from build123d import *

# Parameters (mm, degrees)
BOSS_EXTRUDE1_DEPTH  = 3
M3_CLEARANCE_HOLE1_D = 3.4
CUT_EXTRUDE1_DEPTH   = 10


with BuildPart() as part:
    # Sketch1 → Boss-Extrude1 (new body)
    with BuildSketch(Plane.XY):
        with BuildLine():
            Line((-93.536600288, 73.798841742), (22.52665856, 73.798841742))
            ThreePointArc((22.52665856, 73.798841742), (29.597726372, 76.72777393), (32.52665856, 83.798841742))
            Line((32.52665856, 83.798841742), (32.52665856, 133.798841742))
            ThreePointArc((32.52665856, 133.798841742), (29.597726372, 140.869909554), (22.52665856, 143.798841742))
            Line((22.52665856, 143.798841742), (-93.536600288, 143.798841742))
            ThreePointArc((-93.536600288, 143.798841742), (-100.6076681, 140.869909554), (-103.536600288, 133.798841742))
            Line((-103.536600288, 133.798841742), (-103.536600288, 83.798841742))
            ThreePointArc((-103.536600288, 83.798841742), (-100.6076681, 76.72777393), (-93.536600288, 73.798841742))
        make_face()
        Polygon((7.241251279, 79.113754803), (7.241251279, 115.298841742), (25.200464445, 115.298841742), (25.200464445, 141.298841742), (-63.686125174, 141.298841742), (-63.686125174, 139.298841742), (-98, 139.298841742), (-98, 79.113754803), align=None, mode=Mode.SUBTRACT)
    extrude(amount=BOSS_EXTRUDE1_DEPTH)

    # M3 Clearance Hole1 (through all)
    with Locations(Plane(origin=(0, 0, 0), x_dir=(-1, 0, 0), z_dir=(0, 0, -1))):
        with Locations((-28.497536526, 136.798841742), (-28.497536526, 81.798841742)):
            Hole(M3_CLEARANCE_HOLE1_D / 2)

    # Sketch2 → Cut-Extrude1 (cut)
    with BuildSketch(Plane.XY.offset(3)):
        with BuildLine():
            Line((-98, 111.232980273), (-100.276015927, 111.232980273))
            Line((-100.276015927, 111.232980273), (-100.276015927, 110.181279495))
            ThreePointArc((-100.276015927, 110.181279495), (-100.885260547, 108.11074669), (-101.110575194, 110.257259772))
            Line((-101.110575194, 110.257259772), (-101.110575194, 111.232980273))
            Line((-101.110575194, 111.232980273), (-103.536600288, 111.232980273))
            Line((-103.536600288, 111.232980273), (-103.536600288, 155.169137996))
            Line((-103.536600288, 155.169137996), (37.520914888, 146.495442913))
            Line((37.520914888, 146.495442913), (36.419995989, 128.591552724))
            Line((36.419995989, 128.591552724), (32.52665856, 128.591552724))
            Line((32.52665856, 128.591552724), (29.357018022, 128.591552724))
            Line((29.357018022, 128.591552724), (29.357018022, 126.79555932))
            ThreePointArc((29.357018022, 126.79555932), (28.609769319, 124.402587901), (28.09640217, 126.856390462))
            Line((28.09640217, 126.856390462), (28.09640217, 128.591552724))
            Line((28.09640217, 128.591552724), (25.200464445, 128.591552724))
            Line((25.200464445, 128.591552724), (-98, 111.232980273))
        make_face()
    extrude(amount=-CUT_EXTRUDE1_DEPTH, mode=Mode.SUBTRACT)


solid = part.part
Input: part model. Units: mm. Frame: model coordinates. A direction names the side the tool comes from. Give positions to 0.01 mm unless a question says otherwise; leave off trailing zeros. Write each loop counter-clockwise with the first axis right and the second up, starting at its lowest first coordinate (ties: lowest second). Pieces come first, ordered by that corner, then holes.
Q1. Set-up query: faces 1 (the face through (-103.537, 98, 1)), 2 (the face through (-99, 111.233, 2)), 3 (the face through (-46, 79.114, 1)). Return all of +Z, -Z, +X, -X, +Y, -Y with unobstructed straight access to the full face (end or side cutting, diameter ignored); none if empty.
Q2. First-contact query: P1, Ø0.5, axis at y = 127, z = 2, coming from the -X side; P2, Ø0.7, axis at x = -99, z = 1.5, coming from the +Y side. Flat tips, straight axial feed; report the tip coordinate or a pass-through.
Q3. Section C-C, the plane y = 114. Output: boundary loops of the cut face in (x, z), plus the area to 3 significant figures.
Q4. Pull-direction query (Y, two-part tool) for faces 4 (the face through (31, 128.592, 2)), 5 (the face through (29.411, 83.232, 1.521)), 6 (the face through (7.241, 97, 1)); classes: pulls with the +Y half, pulls with the -Y half, needs draft (parallel to the pull), parting line crosses it, or undercut.
Q5. Section D-D, the plane x = -44. Output: boundary loops of the cut face in (y, z), plus the area to 3 significant figures.
Q6. Material intervals for probe 1 along X at (y, z) = (97, 0.6); probe 2 along X at (y, z) = (122, 1.65); probe 3 along Y at (x, z) = (-12, 2.8), sorted ascending.
Q7. Section B-B, the plane z = 1.45. Output: boundary loops of the cut face in (x, y).
Q8. Section A-A, the plane y = 95.5. Output: boundary loops of the cut face in (x, z).
Filled in:
1. face 1: +Z, -Z, -X, +Y, -Y
1. face 2: +Z, -Z, -X, +Y
1. face 3: +Z, -Z, +Y
2. P1: stops at x = 25.2
2. P2: stops at y = 111.23
3. outline: (7.24, 0) - (32.53, 0) - (32.53, 3) - (7.24, 3) - close
3. area: 75.9 mm2
4. face 4: pulls with the +Y half
4. face 5: undercut
4. face 6: needs draft
5. outline: (73.8, 0) - (79.11, 0) - (79.11, 3) - (73.8, 3) - close
5. area: 15.9 mm2
6. probe 1: x = -103.54 to -98, 7.24 to 32.53
6. probe 2: x = 25.2 to 32.53
6. probe 3: y = 73.8 to 79.11
7. outline: (-103.54, 83.8) arc R10 ccw to (-93.54, 73.8) - (22.53, 73.8) arc R10 ccw to (32.53, 83.8) - (32.53, 128.59) - (29.36, 128.59) - (29.36, 126.8) arc R1.3 cw (long way) to (28.1, 126.86) - (28.1, 128.59) - (25.2, 128.59) - (25.2, 115.3) - (7.24, 115.3) - (7.24, 79.11) - (-98, 79.11) - (-98, 111.23) - (-100.28, 111.23) - (-100.28, 110.18) arc R1.1 cw (long way) to (-101.11, 110.26) - (-101.11, 111.23) - (-103.54, 111.23) - close; hole circle Ø3.4 at (28.5, 81.8)
8. outline: (-103.54, 0) - (-98, 0) - (-98, 3) - (-103.54, 3) - close; (7.24, 0) - (32.53, 0) - (32.53, 3) - (7.24, 3) - close
